from build123d import *

# Parameters (mm, degrees)
SKETCH_1_R               = 12.5
EXTRUDE_1_DEPTH          = 230
SKETCH_2_R               = 3
CUT_EXTRUDE_1_DEPTH      = 20
PATTERN_CIRCULAR_1_COUNT = 3
MIRROR_1_COPY_1_SKETCH_R = 3
MIRROR_1_COPY_1_DEPTH    = 20
MIRROR_1_COPY_2_SKETCH_R = 3
MIRROR_1_COPY_2_DEPTH    = 20


with BuildPart() as part:
    # 草图1 → 凸台-拉伸1 (new body)
    with BuildSketch(Plane(origin=(0, 0, 0), x_dir=(0, 0, -1), z_dir=(1, 0, 0))):
        Circle(SKETCH_1_R)
    extrude(amount=EXTRUDE_1_DEPTH)

    # 草图2 → 切除-拉伸1 (cut)
    with BuildSketch(Plane(origin=(230, 0, 0), x_dir=(0, 0, -1), z_dir=(1, 0, 0))):
        with Locations((0, 8)):
            Circle(SKETCH_2_R)
    cut_extrude_1 = extrude(amount=-CUT_EXTRUDE_1_DEPTH, mode=Mode.SUBTRACT)

    # 阵列(圆周)1: 切除-拉伸1 ×3 about axis
    pattern_circular_1_axis = Axis((0, 0, 0), (1, 0, 0))
    for i in range(1, PATTERN_CIRCULAR_1_COUNT):
        add(cut_extrude_1.rotate(pattern_circular_1_axis, i * 360 / PATTERN_CIRCULAR_1_COUNT), mode=Mode.SUBTRACT)

    # 镜向1: 切除-拉伸1 across plane
    add(cut_extrude_1.mirror(Plane(origin=(115, 0, 0), x_dir=(0, 0, 1), z_dir=(1, 0, 0))), mode=Mode.SUBTRACT)

    # 镜向1 copy 1 sketch → 镜向1 copy 1 (cut)
    with BuildSketch(Plane(origin=(0, 0, 0), x_dir=(0, 0.8660254037844387, 0.4999999999999998), z_dir=(-1, 0, 0))):
        with Locations((0, -8)):
            Circle(MIRROR_1_COPY_1_SKETCH_R)
    extrude(amount=-MIRROR_1_COPY_1_DEPTH, mode=Mode.SUBTRACT)

    # 镜向1 copy 2 sketch → 镜向1 copy 2 (cut)
    with BuildSketch(Plane(origin=(0, 0, 0), x_dir=(0, -0.8660254037844384, 0.5000000000000004), z_dir=(-1, 0, 0))):
        with Locations((0, -8)):
            Circle(MIRROR_1_COPY_2_SKETCH_R)
    extrude(amount=-MIRROR_1_COPY_2_DEPTH, mode=Mode.SUBTRACT)


solid = part.part
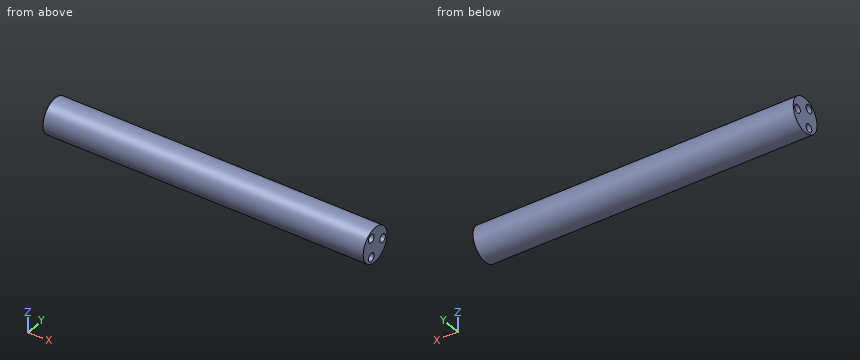
Source: CAD feature listing. Evaluate the final solid. Frame: model axes, mm. Coordinates: 2 decimals unless noted, no trailing zeros. Loops run counter-clockwise (first coordinate to the right, second up) from the corner with the lowest first, then second, coordinate; pieces in that order, holes last. Notation, with made-up numbers: M 76.25,-29.75 L 102.25,-29.75 A30 cw 102.25,3.25 Z; hole C 75.25,47 d3. An arc over 180 degrees is marked long. Answer in a Markdown table with one row per item.
Q1. First-contact query: pin 1 (5 mm diameter, centred on y = -4, z = 6.93, fed in from -X); pin 2 (5 mm diameter, centred on x = 33, z = -5.5, fed in from -Y); pin 3 (1.8 mm diameter, centred on y = -4.5, z = 6, fed in from +X). Flat tips, straight axial feed; report the tip coordinate or a pass-through.
Answers below:
| item | result |
|---|---|
| pin 1 | stops at x = 20 |
| pin 2 | stops at y = -12.13 |
| pin 3 | stops at x = 210 |
Q2. Section A-A on z = 0. Return the cut outline in (x, y).
Answers below:
| item | result |
|---|---|
| outline | M 0,-12.5 L 230,-12.5 L 230,5 L 210,5 L 210,11 L 230,11 L 230,12.5 L 0,12.5 L 0,11 L 20,11 L 20,5 L 0,5 Z |
Q3. Section D-D on x = 215.5. Return the cut outline in (y, z), plus the area to 3 significant figures.
Answers below:
| item | result |
|---|---|
| outline | C 0,0 d25; hole C -4,-6.93 d6; hole C -4,6.93 d6; hole C 8,0 d6 |
| area | 406 mm^2 |
Q4. Ray query, probe 1 along Z at (x, y) = (21.5, 1); probe 2 along X at (y, z) = (10.5, -0.75); probe 3 along Y at (x, z) = (10.25, 0). Return the intervals inside material, ascending. Write a range as from..to.
Answers below:
| item | result |
|---|---|
| probe 1 | z = -12.46..12.46 |
| probe 2 | x = 20..210 |
| probe 3 | y = -12.5..5, 11..12.5 |
Q5. Section C-C on x = 120. Return the cut outline in (y, z).
Answers below:
| item | result |
|---|---|
| outline | C 0,0 d25 |
Q6. Section B-B on y = 8. Return the cut outline in (x, z).
Answers below:
| item | result |
|---|---|
| outline | M 0,-9.6 L 230,-9.6 L 230,-3 L 210,-3 L 210,3 L 230,3 L 230,9.6 L 0,9.6 L 0,3 L 20,3 L 20,-3 L 0,-3 Z |
